from build123d import *

# Parameters (mm, degrees)
F1_DEPTH = 9.525
F2_DEPTH = 9.525
F3_D     = 4.7625
F4_D     = 4.7625
F5_D     = 4.7625
F6_D     = 4.7625


with BuildPart() as f1:
    # F0 (on Front) → F1 (new body)
    with BuildSketch(Plane.XZ):
        Polygon((211.2021158695, -16.6006076694), (-185.6728841305, -16.6006076694), (-236.4728841305, -73.7506076694), (-185.6728841305, -73.7506076694), (-93.5978841305, -73.7506076694), (119.1271158695, -73.7506076694), (211.2021158695, -73.7506076694), (262.0021158695, -73.7506076694), align=None)
    extrude(amount=F1_DEPTH)

    # F0 (on Front) → F2 (join)
    with BuildSketch(Plane.XZ):
        Polygon((211.2021158695, -16.6006076694), (-185.6728841305, -16.6006076694), (-236.4728841305, -73.7506076694), (-185.6728841305, -73.7506076694), (-93.5978841305, -73.7506076694), (119.1271158695, -73.7506076694), (211.2021158695, -73.7506076694), (262.0021158695, -73.7506076694), align=None)
    extrude(amount=F2_DEPTH)

    # F3 (through all)
    with Locations(Plane(origin=(0, 0, 0), x_dir=(1, 0, 0), z_dir=(0, 1, 0))):
        with Locations((114.9996158695, 45.1756076694)):
            Hole(F3_D / 2)

    # F4 (through all)
    with Locations(Plane(origin=(0, 0, 0), x_dir=(1, 0, 0), z_dir=(0, 1, 0))):
        with Locations((-89.4703841305, 45.1756076694)):
            Hole(F4_D / 2)

    # F5 (through all)
    with Locations(Plane(origin=(0, 0, 0), x_dir=(1, 0, 0), z_dir=(0, 1, 0))):
        with Locations((206.4396158695, 45.1756076694)):
            Hole(F5_D / 2)

    # F6 (through all)
    with Locations(Plane(origin=(0, 0, 0), x_dir=(1, 0, 0), z_dir=(0, 1, 0))):
        with Locations((-180.9103841305, 45.1756076694)):
            Hole(F6_D / 2)


solid = f1.part
The listing builds one solid part. Answer for the finished solid, in the listing's coordinates (mm). Round coordinates to 2 decimals unless told otherwise and drop trailing zeros. Write each loop counter-clockwise with the first axis right and the second up, starting at its lowest first coordinate (ties: lowest second). Pieces come first, ordered by that corner, then holes. Notation, with made-up numbers: M -8.5,-31 L 20.5,-31 A34 ccw 20.5,0 Z; hole C -16.5,70 d10. An arc over 180 degrees is marked long. Write each question's results on one line, items separated by ' | '. Start each with the question number.
Item 1: Find section A-A on y = -4.5. Write down the section's boundary in (x, z).
Item 2: Straight lines are drawn through the part: probe 1 along X at (y, z) = (-6, -43.5); probe 2 along X at (y, z) = (-1.25, -45); probe 3 along Z at (x, y) = (222, -2.75). For each, find the intervals that lie inside material, in ascending order.
Item 3: The mould has two halves that part along Z. Classify faces 1 (the flat face through (-210.72, -4.7, -44.78)), 2 (the flat face through (9, 0, -45)), 3 (the flat face through (9, -5, -73.751)): +Z half, -Z half, draft (parallel to the pull), parting line (faces both ways), or undercut.
Item 4: Given pin 1 Ø4 at (y, z) = (-6, -64) entering from -X; pin 2 Ø5 at (y, z) = (-2.5, -55.5) entering from +X; pin 3 Ø1 at (y, z) = (-7, -36.5) entering from +X, each flat-ended and moving along its own axis, determine where each tip first touches the part or whether it passes through.
Item 5: Find section B-B on z = -57.5. Write down the section's boundary in (x, y) (3 decimals), and give its area (3 significant figures).
Answer block:
1) outline: M -236.47,-73.75 L 262,-73.75 L 211.2,-16.6 L -185.67,-16.6 Z; hole C -180.91,-45.18 d4.76; hole C -89.47,-45.18 d4.76; hole C 115,-45.18 d4.76; hole C 206.44,-45.18 d4.76
2) probe 1: x = -209.58 to -182.6, -179.22 to -91.16, -87.78 to 113.31, 116.69 to 204.75, 208.13 to 235.11 | probe 2: x = -210.92 to -183.29, -178.54 to -91.85, -87.1 to 112.62, 117.37 to 204.06, 208.81 to 236.45 | probe 3: z = -73.75 to -28.75
3) face 1: +Z half | face 2: draft | face 3: -Z half
4) pin 1: stops at x = -229.58 | pin 2: stops at x = 248 | pin 3: stops at x = 229.33
5) outline: M -222.028,-9.525 L 247.557,-9.525 L 247.557,0 L -222.028,0 Z | area: 4,470 mm²
